Model file for the job. Use its own axes, mm. A direction names the side the tool comes from. Coordinates: 2 decimals unless noted, no trailing zeros. Loops run counter-clockwise (first coordinate to the right, second up) from the corner with the lowest first, then second, coordinate; pieces in that order, holes last. Notation, with made-up numbers: (-31, -32) -> (0, -32) arc R18 ccw to (0, -21) -> close; hole circle Ø6 at (-13, 38). An arc over 180 degrees is marked (long way). Use one line per item in the form item = value.
Autodesk Inventor part; units mm, degrees
ref_plane "Work Plane1" through (0, 0, 5) normal (0, 0, 1) x (1, 0, 0)
ref_plane "Work Plane2" through (0, 0, 5) normal (0, 0, -1) x (-1, 0, 0)
ref_plane "Work Plane3" through (1.5, 7.5, 45) normal (0, 0.5, 0.866) x (-1, 0, 0)
sketch "Sketch1" plane through (0, 0, 0) normal (0, 0, 1) x (1, 0, 0)
  circle A0 centre (0, 0) radius 7.5
  dimension "d0" = 15
ref_plane "Work Plane1" through (0, 0, 5) normal (0, 0, 1) x (1, 0, 0)
sketch "Sketch2" plane through (0, 0, 5) normal (0, 0, 1) x (1, 0, 0)
  circle A0 centre (0, 0) radius 5
  dimension "d4" = 10
loft "Loft1" add profiles "Sketch1", "Sketch2"
sketch "Sketch3" plane through (0, 0, 5) normal (0, 0, 1) x (1, 0, 0)
  circle A0 centre (0, 0) radius 5
  dimension "d9" = 10
extrude "Extrusion2" add sketch "Sketch3" along normal blind 15
sketch "Sketch4" plane through (0, 0, 20) normal (0, 0, 1) x (1, 0, 0)
  line L0 (5, 0) -> (-5, 0)
  arc A0 (-5, 0) -> (5, 0) centre (0, 0) ccw
revolve "Revolution1" add sketch "Sketch4" angle 180 about axis through (5, 0, 20) along (-1, 0, 0)
ref_plane "Work Plane2" through (0, 0, 5) normal (0, 0, -1) x (-1, 0, 0)
sketch "Sketch6" plane through (0, 0, 5) normal (0, 0, -1) x (-1, 0, 0)
  line L0 (-1.5, 7.5) -> (1.5, 7.5)
  line L1 (1.5, -2.5) -> (0, -7.5)
  line L2 (0, -7.5) -> (-1.5, -2.5)
  line L3 (1.5, 7.5) -> (1.5, -2.5)
  line L4 (-1.5, -2.5) -> (-1.5, 7.5)
  line L5 (0.9, -4.5) -> (-1.5, 7.5) construction
  line L6 (-0.9, -4.5) -> (1.5, 7.5) construction
  point P0 (0, 0)
  point P1 (0, 7.5)
  point P2 (0, 0)
  dimension "d14" = 3
extrude "Extrusion3" add sketch "Sketch6" against normal blind 40
ref_plane "Work Plane3" through (1.5, 7.5, 45) normal (0, 0.5, 0.866) x (-1, 0, 0)
sketch "Sketch7" plane through (1.5, 7.5, 45) normal (0, 0.5, 0.866) x (-1, 0, 0)
  line L0 (0, 16.105) -> (3, 16.105)
  line L1 (3, 16.105) -> (3, -7.3572)
  line L2 (3, -7.3572) -> (0, -7.3572)
  line L3 (0, -7.3572) -> (0, 16.105)
  line L4 (0, 16.105) -> (3, -7.3572) construction
  line L5 (3, 16.105) -> (0, -7.3572) construction
  point P0 (1.5, -16.0048)
  point P1 (1.5, 4.3739)
  dimension "d19" = 23.4622
extrude "Extrusion4" cut sketch "Sketch7" against normal blind 7.5
properties part number "Cutter"
Q1. Band-saw the part on A-A, the plane z = 25.5. Write the cut outline in (x, y), and give its area (3 significant figures).
Result:
outline = (-1.5, -2.5) -> (0, -7.5) -> (1.5, -2.5) -> (1.5, 7.5) -> (-1.5, 7.5) -> close
area = 37.5 mm2
Q2. Wall check: line 1 along X through (y, z) = (2, 25); line 2 along Z through (x, y) = (0.5, 5.5); line 3 along Z through (x, y) = (1, 7.25). Give the ranges that are in metal, low to high.
Result:
line_1 = -1.5 to 1.5
line_2 = 0 to 3.95, 5 to 37.49
line_3 = 0 to 0.36, 5 to 36.48
Q3. Pin check, flat tips, straight feed: pin 1 Ø1 at (y, z) = (-2.5, 40) entering from +X; pin 2 Ø4 at (x, z) = (-4.5, 10.5) entering from -Y; pin 3 Ø3 at (y, z) = (4, 21) entering from +X. Stop position of each tip, or through.
Result:
pin_1 = 1.5
pin_2 = -4.33
pin_3 = 4.26
Q4. Mould opens along Z. For faces 5 (the face through (0, -6, 5)), 6 (the face through (0, 0, 0)), 7 (the face through (0, 7.5, 20)) say: released by +Z, released by -Z, zero draft, split by the parting line, or undercut.
Result:
face_5 = undercut
face_6 = released by -Z
face_7 = zero draft
Q5. Band-saw the part on B-B, the plane z = 6. Write the cut outline in (x, y).
Result:
outline = (-1.5, 4.77) arc R5 ccw to (-0.77, -4.94) -> (0, -7.5) -> (0.77, -4.94) arc R5 ccw to (1.5, 4.77) -> (1.5, 7.5) -> (-1.5, 7.5) -> close
Q6. Which spindle directions (+Z, -Z, +X, -X, +Y, -Y) get a long thin tool onto all of the face, cutting with end or side? Do faces 1 (the face through (-5, 0, 12)), 2 (the face through (5, 0, 12)), 3 (the face through (-0.6, -5.5, 29.2)), 4 (the face through (0.573, -5.591, 29.163)). Say none if no direction does.
Result:
face_1 = +Z, -X
face_2 = +Z, +X
face_3 = +Z, -X, -Y
face_4 = +Z, +X, -Y
